Geometry: see drawing. Coordinates: mm, zero at the bounding-box minimum. A direction names the side the tool comes from. Coordinates: 2 decimals unless noted, no trailing zeros. Write each loop counter-clockwise with the first axis right and the second up, starting at its lowest first coordinate (ties: lowest second). Pieces come first, ordered by that corner, then holes. Notation, with made-up numbers: M 20.25,17.5 L 70.25,17.5 A11 cw 70.25,25.5 Z; hole C 44,66 d2. An arc over 180 degrees is marked long. Answer as CSV lines item,"result". Start each with the question number.
1. Reachability of the marked faces 1, 2, 3, 4 and 5 from +Z, -Z, +X, -X, +Y, -Y: full face, straight path, thin tool, end or side. Return the list, or none.
2. Section D-D on x = 48. Return the cut outline in (y, z), plus the area to 3 significant figures.
3. Contact query for flat-ended pins moving along their axis: pin 1 Ø5 at (x, y) = (49, 83.5) entering from -Z; pin 2 Ø5.5 at (x, z) = (6.35, 31.75) entering from -Y; pin 3 Ø8 at (x, y) = (27, 33.5) entering from -Z (1 decimal). Output: stop coordinate, or through.
4. Section C-C on y = 42. Return the cut outline in (x, z), plus the area to 3 significant figures.
5. Section A-A on z = 6.35. Return the cut outline in (x, y).
6. Line query: probe 1 along Z at (x, y) = (57, 116); probe 2 along Z at (x, y) = (31.75, 116). Output: solid intervals per line, ascending. Write a range as [from, to].
7. Section B-B on x = 57.15. Return the cut outline in (y, z), plus the area to 3 significant figures.
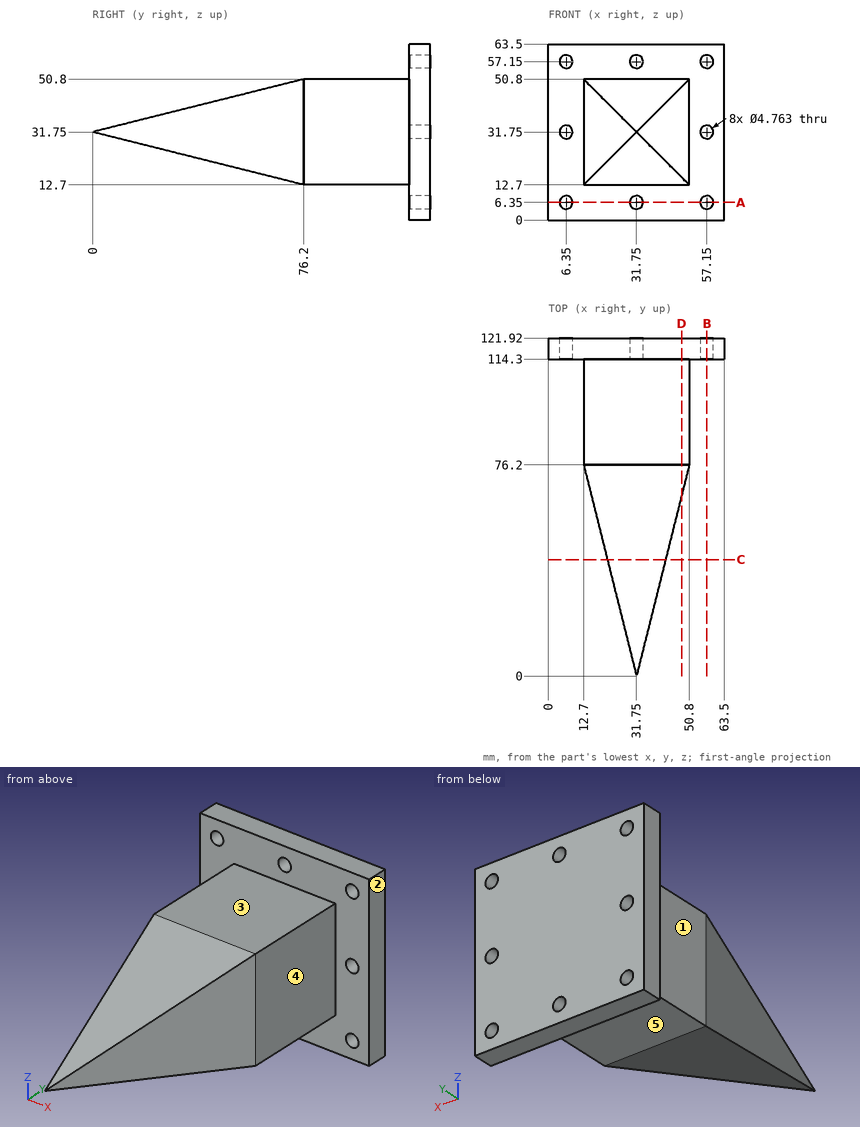
Values:
1,face 1,"+Z, -Z, -X, -Y"
1,face 2,"+Z, -Z, +X, +Y, -Y"
1,face 3,"+Z, +X, -X, -Y"
1,face 4,"+Z, -Z, +X, -Y"
1,face 5,"-Z, +X, -X, -Y"
2,outline,"M 65,15.5 L 76.2,12.7 L 114.3,12.7 L 114.3,0 L 121.92,0 L 121.92,63.5 L 114.3,63.5 L 114.3,50.8 L 76.2,50.8 L 65,48 Z"
2,area,"2,330 mm²"
3,pin 1,"z = 12.7"
3,pin 2,"y = 114.3"
3,pin 3,"z = 22.4"
4,outline,"M 21.25,21.25 L 42.25,21.25 L 42.25,42.25 L 21.25,42.25 Z"
4,area,"441 mm²"
5,outline,"M 0,114.3 L 3.97,114.3 L 3.97,121.92 L 0,121.92 Z; M 8.73,114.3 L 29.37,114.3 L 29.37,121.92 L 8.73,121.92 Z; M 34.13,114.3 L 54.77,114.3 L 54.77,121.92 L 34.13,121.92 Z; M 59.53,114.3 L 63.5,114.3 L 63.5,121.92 L 59.53,121.92 Z"
6,probe 1,"[0, 3.97], [8.73, 29.37], [34.13, 54.77], [59.53, 63.5]"
6,probe 2,"[0, 3.97], [8.73, 54.77], [59.53, 63.5]"
7,outline,"M 114.3,0 L 121.92,0 L 121.92,3.97 L 114.3,3.97 Z; M 114.3,8.73 L 121.92,8.73 L 121.92,29.37 L 114.3,29.37 Z; M 114.3,34.13 L 121.92,34.13 L 121.92,54.77 L 114.3,54.77 Z; M 114.3,59.53 L 121.92,59.53 L 121.92,63.5 L 114.3,63.5 Z"
7,area,"375 mm²"
